Can you work these out from the model? Positions are in its coordinate system, mm. Face numbers are marked on the shaded views. A direction names the side the tool comes from. Give positions to 0.01 mm unless a question says otherwise; leave off trailing zeros. Write each loop counter-clockwise with the first axis right and the second up, starting at its lowest first coordinate (ties: lowest second). Pieces come first, ordered by that corner, then holes. Notation, with made-up numbers: (41.25, -26.5) - (63.25, -26.5) arc R23 cw to (63.25, 2.5) - close; hole circle Ø9 at (-9, 6). An arc over 180 degrees is marked (long way). Return JSON: item names as keys, results as strings. Group by question number.
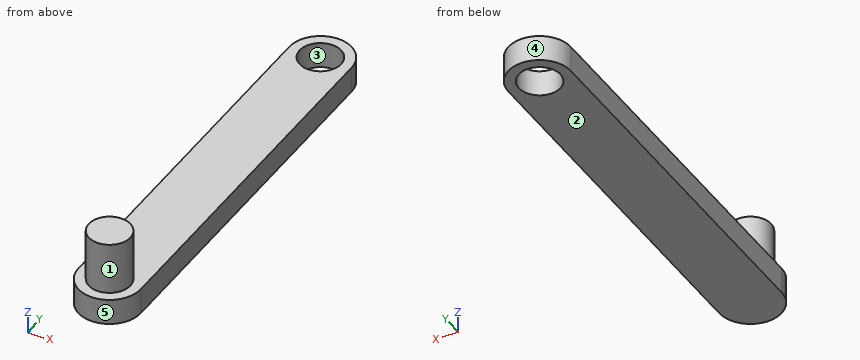
from build123d import *

# Parameters (mm, degrees)
SKETCH1_R           = 4
BOSS_EXTRUDE1_DEPTH = 5
SKETCH2_R           = 4
BOSS_EXTRUDE2_DEPTH = 10


with BuildPart() as part:
    # Sketch1 → Boss-Extrude1 (new body)
    with BuildSketch(Plane.XY):
        with BuildLine():
            Line((-6, -36), (-6, 36))
            ThreePointArc((-6, 36), (0, 42), (6, 36))
            Line((6, 36), (6, -36))
            ThreePointArc((6, -36), (0, -42), (-6, -36))
        make_face()
        with Locations((0, 36)):
            Circle(SKETCH1_R, mode=Mode.SUBTRACT)
    extrude(amount=BOSS_EXTRUDE1_DEPTH)

    # Sketch2 → Boss-Extrude2 (add)
    with BuildSketch(Plane.XY.offset(5)):
        with Locations((0, -36)):
            Circle(SKETCH2_R)
    extrude(amount=BOSS_EXTRUDE2_DEPTH)


solid = part.part
1) I need wall thicknesses on line 1 along Y through (x, z) = (0, 2.2); line 2 along Z through (x, y) = (2.5, -20.5); line 3 along X through (y, z) = (37, 2.75). Which ranges of each line are inside material? Lowest first, please.
2) Imagine slicing it at C-C, the plane y = 9. Write out the boundary of the cut face in (x, z).
3) Imagine slicing it at B-B, the plane z = 2.25. Write out the boundary of the cut face in (x, y).
4) Imagine slicing it at A-A, the plane x = 0. Write out the boundary of the cut face in (y, z), and give its area (3 significant figures).
5) We'd pull the mould along Y, two halves only. Please class the marked faces 3, 4 and 5: pulls with the +Y half, pulls with the -Y half, needs draft (parallel to the pull), parting line crosses it, or undercut.
6) Will these pins go through, and if not, where does the flat tip stop? pin 1 Ø1.5 at (x, z) = (0.5, 13) entering from +Y; pin 2 Ø1 at (x, y) = (-1.5, -14) entering from -Z; pin 3 Ø1.5 at (y, z) = (27, 6.5) entering from -X; pin 4 Ø2 at (x, z) = (-3, 10) entering from -Y.
7) On a 3-axis mill with a long thin cutter (end or side, diameter ignored), from which of +Z, -Z, +X, -X, +Y, -Y can I reach the whole of each face in a straight line? I mean the marked faces 1 and 2. Say none if no direction works.
8) Imagine slicing it at D-D, the plane z = 10. Write out the boundary of the cut face in (x, y).
Resolved:
{
 "1": {"line 1": "-42 to 32, 40 to 42", "line 2": "0 to 5", "line 3": "-5.92 to -3.87, 3.87 to 5.92"},
 "2": {"outline": "(-6, 0) - (6, 0) - (6, 5) - (-6, 5) - close"},
 "3": {"outline": "(-6, -36) arc R6 ccw to (6, -36) - (6, 36) arc R6 ccw to (-6, 36) - close; hole circle Ø8 at (0, 36)"},
 "4": {"outline": "(-42, 0) - (32, 0) - (32, 5) - (-32, 5) - (-32, 15) - (-40, 15) - (-40, 5) - (-42, 5) - close; (40, 0) - (42, 0) - (42, 5) - (40, 5) - close", "area": "460 mm^2"},
 "5": {"face 3": "undercut", "face 4": "pulls with the +Y half", "face 5": "pulls with the -Y half"},
 "6": {"pin 1": "y = -32", "pin 2": "z = 0", "pin 3": "through", "pin 4": "y = -39.46"},
 "7": {"face 1": "+Z", "face 2": "-Z, +X, -X, +Y, -Y"},
 "8": {"outline": "circle Ø8 at (0, -36)"}
}
